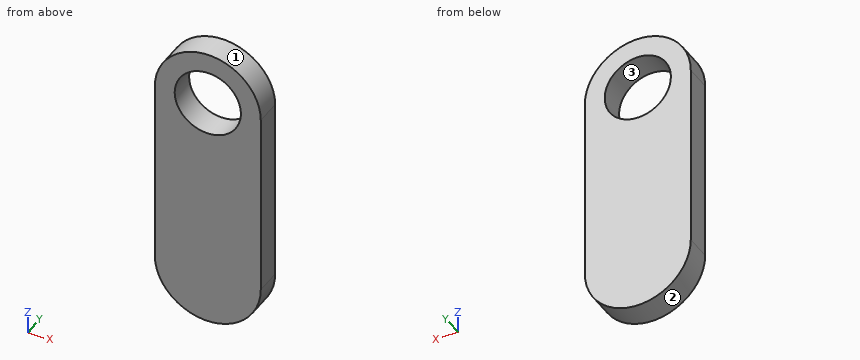
Autodesk Inventor part; units mm, degrees
ref_plane "YZ Plane" through (0, 0, 0) normal (1, 0, 0) x (0, 1, 0)
ref_plane "XZ Plane" through (0, 0, 0) normal (0, 1, 0) x (-1, 0, 0)
ref_plane "XY Plane" through (0, 0, 0) normal (0, 0, 1) x (1, 0, 0)
sketch "Sketch1" plane through (0, 0, 0) normal (0, 1, 0) x (-1, 0, 0)
  line L0 (0, 7) -> (0, -7) construction
  line L1 (-4, 7) -> (-4, -7)
  line L2 (4, -7) -> (4, 7)
  arc A0 (4, 7) -> (-4, 7) centre (0, 7) ccw
  arc A1 (-4, -7) -> (4, -7) centre (0, -7) ccw
  circle A2 centre (0, 7) radius 2.5
  point P0 (0, 0)
  point P1 (0, 0)
  point P2 (0, -11)
  dimension "d0" = 8
  dimension "d1" = 18
  dimension "d2" = 5
extrude "Extrusion1" add sketch "Sketch1" along normal blind 2
properties part number "servo-arm"
Read the model definition and answer for the solid it produces. Units are mm, in the model's axes. Face numbers are marked on the shaded views. Give positions to 0.01 mm unless a question says otherwise; leave off trailing zeros. Loops run counter-clockwise (first coordinate to the right, second up) from the corner with the lowest first, then second, coordinate; pieces in that order, holes last.
Item 1: The part is cut by section C-C (x = 1.25). Write down the section's boundary in (y, z).
Item 2: The part is cut by section A-A (x = 0). Write down the section's boundary in (y, z).
Item 3: This flat-tipped pin is pushed along its axis until it touches: pin 1 Ø1 at (x, y) = (1.5, 1.5) entering from -Z. Where does it stop, or does it pass through?
Item 4: The part is cut by section B-B (y = 0.35). Write down the section's boundary in (x, z).
Item 5: The mould has two halves that part along Z. Classify the marked faces 1, 2 and 3: released by +Z, released by -Z, zero draft, split by the parting line, or undercut.
Item 6: Find the intervals of material crossed by line 1 along Z through (x, y) = (0, 0.7); line 2 along Z through (x, y) = (-2, 1.75); line 3 along X through (y, z) = (1.8, 8.75), in increasing order.
Item 7: The part is cut by section D-D (z = -9.25). Write down the section's boundary in (x, y).
Taken from the geometry:
1. outline: (0, -10.8) - (2, -10.8) - (2, 4.83) - (0, 4.83) - close; (0, 9.17) - (2, 9.17) - (2, 10.8) - (0, 10.8) - close
2. outline: (0, -11) - (2, -11) - (2, 4.5) - (0, 4.5) - close; (0, 9.5) - (2, 9.5) - (2, 11) - (0, 11) - close
3. pin 1: stops at z = -10.87
4. outline: (-4, -7) arc R4 ccw to (4, -7) - (4, 7) arc R4 ccw to (-4, 7) - close; hole circle Ø5 at (0, 7)
5. face 1: released by +Z
5. face 2: released by -Z
5. face 3: undercut
6. line 1: z = -11 to 4.5, 9.5 to 11
6. line 2: z = -10.46 to 5.5, 8.5 to 10.46
6. line 3: x = -3.6 to -1.79, 1.79 to 3.6
7. outline: (-3.31, 0) - (3.31, 0) - (3.31, 2) - (-3.31, 2) - close
